Here's how the part is built. I have some questions about the finished solid (model axes, mm). A direction names the side the tool comes from. Coordinates: 2 decimals unless noted, no trailing zeros. Write each loop counter-clockwise with the first axis right and the second up, starting at its lowest first coordinate (ties: lowest second). Pieces come first, ordered by that corner, then holes.
Item 1: If we section it at C-C (y = 73.5): Please give me the cut outline in (x, z), then the cut area to 3 significant figures.
Item 2: If we section it at D-D (y = -6): Please give me the cut outline in (x, z).
Item 3: For faces 5 (the face through (30, 36, 19)), 6 (the face through (13, 52, 19)), 7 (the face through (39.067, 73.541, 13.648)), which set-ups out of +Z, -Z, +X, -X, +Y, -Y let a thin tool reach every point of the face, with its end or its side?
Item 4: I'm going to push flat-ended pins straight in: pin 1 Ø5 at (y, z) = (34, 17.5) entering from -X; pin 2 Ø4 at (x, z) = (38, 19.5) entering from -Y; pin 3 Ø6 at (x, y) = (39, 5.5) entering from -Z. Where does each tip first touch, or does it pass through?
Item 5: If I drill on line 1 (Y direction, x = 33, z = 15); line 2 (Y direction, x = 52.4, z = 18); line 3 (X direction, y = 70.5, z = 9.5), over which ranges is the centre line in solid material (lowest first)?
Item 6: If we section it at B-B (z = 19.75): Count the separate pieces of the cut face and the enclosed holes in it, then the cut area to 3 significant figures.
Item 7: If we section it at A-A (y = 39.5): Please give me the cut outline in (x, z).
Item 8: We'd pull the mould along Y, two halves only. Please class faces 1 (the face through (15, -19, 19)), 2 (the face through (20, 53.43, 18.7)), 3 (the face through (30, -15, 19)), 4 (the face through (35.85, 73, 11)): +Y half, -Y half, draft (parallel to the pull), parting line (faces both ways), or undercut.
from build123d import *

# Parameters (mm, degrees)
SKETCH1_R           = 4
SKETCH1_W           = 10.5
SKETCH1_H           = 11.5
BOSS_EXTRUDE1_DEPTH = 22
CUT_EXTRUDE1_DEPTH  = 14
SKETCH5_W           = 17
SKETCH5_H           = 15.5
SKETCH5_R           = 2.9
CUT_EXTRUDE2_DEPTH  = 2.1
CUT_EXTRUDE3_START  = -2.1
SKETCH4_W           = 17
SKETCH4_H           = 15.5
SKETCH4_R           = 2.9
CUT_EXTRUDE3_DEPTH  = 2.1
CUT_EXTRUDE4_START  = -16.1
CUT_EXTRUDE4_DEPTH  = 14
CUT_EXTRUDE5_DEPTH  = 14
CUT_EXTRUDE6_REACH  = 138.799
CUT_EXTRUDE8_DEPTH  = 1.5


with BuildPart() as part:
    # Sketch1 → Boss-Extrude1 (new body)
    with BuildSketch(Plane.XY):
        with BuildLine():
            Line((0, 13.076696831), (0, 42))
            ThreePointArc((0, 42), (2.928932188, 49.071067812), (10, 52))
            Line((10, 52), (16.5, 52))
            ThreePointArc((16.5, 52), (20.035533906, 53.464466094), (21.5, 57))
            Line((21.5, 57), (21.5, 81.25))
            Line((21.5, 81.25), (39.7, 81.25))
            Line((39.7, 81.25), (39.7, 61.75))
            Line((39.7, 61.75), (35, 61.75))
            ThreePointArc((35, 61.75), (31.464466094, 60.285533906), (30, 56.75))
            Line((30, 56.75), (30, 14))
            ThreePointArc((30, 14), (31.464466094, 10.464466094), (35, 9))
            Line((35, 9), (52.4, 9))
            ThreePointArc((52.4, 9), (61.4, 0), (52.4, -9))
            Line((52.4, -9), (35, -9))
            ThreePointArc((35, -9), (31.464466094, -10.464466094), (30, -14))
            Line((30, -14), (30, -17))
            ThreePointArc((30, -17), (27.071067812, -24.071067812), (20, -27))
            Line((20, -27), (12, -27))
            ThreePointArc((12, -27), (8.464466094, -28.464466094), (7, -32))
            Line((7, -32), (7, -39))
            Line((7, -39), (-9, -39))
            Line((-9, -39), (-9, 0))
            ThreePointArc((-9, 0), (-7.413790239, 5.102520386), (-3.214285714, 8.406447963))
            ThreePointArc((-3.214285714, 8.406447963), (-0.881227645, 10.241963283), (0, 13.076696831))
        make_face()
        Circle(SKETCH1_R, mode=Mode.SUBTRACT)
        with Locations((52.4, 0)):
            Circle(SKETCH1_R, mode=Mode.SUBTRACT)
        with BuildLine():
            Line((42.5, -2.5), (26.5, -2.5))
            ThreePointArc((26.5, -2.5), (26.146446609, -2.353553391), (26, -2))
            Line((26, -2), (26, 5))
            ThreePointArc((26, 5), (26.146446609, 5.353553391), (26.5, 5.5))
            Line((26.5, 5.5), (42.5, 5.5))
            ThreePointArc((42.5, 5.5), (42.853553391, 5.353553391), (43, 5))
            Line((43, 5), (43, -2))
            ThreePointArc((43, -2), (42.853553391, -2.353553391), (42.5, -2.5))
        make_face(mode=Mode.SUBTRACT)
        with BuildLine():
            Line((8, 42), (8, -17))
            ThreePointArc((8, -17), (8.585786438, -18.414213562), (10, -19))
            Line((10, -19), (20, -19))
            ThreePointArc((20, -19), (21.414213562, -18.414213562), (22, -17))
            Line((22, -17), (22, 42))
            ThreePointArc((22, 42), (21.414213562, 43.414213562), (20, 44))
            Line((20, 44), (10, 44))
            ThreePointArc((10, 44), (8.585786438, 43.414213562), (8, 42))
        make_face(mode=Mode.SUBTRACT)
        with Locations((30.6, 73.5)):
            Rectangle(SKETCH1_W, SKETCH1_H, mode=Mode.SUBTRACT)
    extrude(amount=BOSS_EXTRUDE1_DEPTH)

    # Sketch3 → Cut-Extrude1 (cut)
    with BuildSketch(Plane(origin=(0, 0, 0), x_dir=(-1, 0, 0), z_dir=(0, 0, -1))):
        with BuildLine():
            Line((-21.5, 61.75), (-35, 61.75))
            ThreePointArc((-35, 61.75), (-31.464466094, 60.285533906), (-30, 56.75))
            Line((-30, 56.75), (-30, 14))
            ThreePointArc((-30, 14), (-31.464466094, 10.464466094), (-35, 9))
            Line((-35, 9), (-52.4, 9))
            ThreePointArc((-52.4, 9), (-61.4, 0), (-52.4, -9))
            Line((-52.4, -9), (-35, -9))
            ThreePointArc((-35, -9), (-31.464466094, -10.464466094), (-30, -14))
            Line((-30, -14), (-30, -17))
            ThreePointArc((-30, -17), (-27.071067812, -24.071067812), (-20, -27))
            Line((-20, -27), (-12, -27))
            ThreePointArc((-12, -27), (-8.464466094, -28.464466094), (-7, -32))
            Line((-7, -32), (-7, -23.75))
            Line((-7, -23.75), (9, -23.75))
            Line((9, -23.75), (9, 0))
            ThreePointArc((9, 0), (7.413790239, 5.102520386), (3.214285714, 8.406447963))
            ThreePointArc((3.214285714, 8.406447963), (0.881227645, 10.241963283), (0, 13.076696831))
            Line((0, 13.076696831), (0, 42))
            ThreePointArc((0, 42), (-2.928932188, 49.071067812), (-10, 52))
            Line((-10, 52), (-16.5, 52))
            ThreePointArc((-16.5, 52), (-20.035533906, 53.464466094), (-21.5, 57))
            Line((-21.5, 57), (-21.5, 61.75))
        make_face()
    extrude(amount=-CUT_EXTRUDE1_DEPTH, mode=Mode.SUBTRACT)

    # Sketch5 → Cut-Extrude2 (cut)
    with BuildSketch(Plane.ZY.offset(-21.5)):
        with Locations((13.5, 73.5)):
            Rectangle(SKETCH5_W, SKETCH5_H)
        with Locations(Location((12.5, 73.5, 0), (0, 0, 90))):
            Circle(SKETCH5_R, mode=Mode.SUBTRACT)
    extrude(amount=-CUT_EXTRUDE2_DEPTH, mode=Mode.SUBTRACT)

    # Sketch4 → Cut-Extrude3 (cut)
    with BuildSketch(Plane(origin=(39.7, 0, 0), x_dir=(0, 0, -1), z_dir=(1, 0, 0)).offset(CUT_EXTRUDE3_START)):
        with Locations((-13.5, 73.5)):
            Rectangle(SKETCH4_W, SKETCH4_H)
        with Locations(Location((-12.5, 73.5, 0), (0, 0, 90))):
            Circle(SKETCH4_R, mode=Mode.SUBTRACT)
    extrude(amount=CUT_EXTRUDE3_DEPTH, mode=Mode.SUBTRACT)

    # Sketch6 → Cut-Extrude4 (cut)
    with BuildSketch(Plane.ZY.offset(-21.5).offset(CUT_EXTRUDE4_START)):
        Polygon((12.5, 81.25), (14.5, 79.25), (22, 79.25), (22, 81.25), align=None)
        Polygon((12.5, 65.75), (14.5, 67.75), (22, 67.75), (22, 65.75), align=None)
    extrude(amount=CUT_EXTRUDE4_DEPTH, mode=Mode.SUBTRACT)

    # Sketch7 → Cut-Extrude5 (cut)
    with BuildSketch(Plane.XY.offset(22)):
        Polygon((25.35, 81.25), (35.85, 81.25), (35.85, 65.75), (39.7, 65.75), (39.7, 65.25), (21.5, 65.25), (21.5, 65.75), (25.35, 65.75), align=None)
    extrude(amount=-CUT_EXTRUDE5_DEPTH, mode=Mode.SUBTRACT)

    # Cut-Extrude6: up to this face of the body (flat: up to its plane)
    cut_extrude6_end = Plane(part.part.faces().sort_by_distance((22.55, 65.75, 6.5))[0])
    # Sketch8 → Cut-Extrude6 (cut, up to the picked face)
    with BuildSketch(Plane(origin=(0, 81.25, 0), x_dir=(1, 0, 0), z_dir=(0, 1, 0)), mode=Mode.PRIVATE) as cut_extrude6_sk1:
        Polygon((21.5, -12.5), (23.1, -15.4), (21.5, -15.4), align=None)
    cut_extrude6_tool1 = split(extrude(cut_extrude6_sk1.sketch, amount=-CUT_EXTRUDE6_REACH, mode=Mode.PRIVATE), bisect_by=cut_extrude6_end, keep=Keep.BOTH, mode=Mode.PRIVATE)
    # Sketch8 → Cut-Extrude6 (cut, up to the picked face)
    with BuildSketch(Plane(origin=(0, 81.25, 0), x_dir=(1, 0, 0), z_dir=(0, 1, 0)), mode=Mode.PRIVATE) as cut_extrude6_sk2:
        Polygon((39.7, -15.4), (38.1, -15.4), (39.7, -12.5), align=None)
    cut_extrude6_tool2 = split(extrude(cut_extrude6_sk2.sketch, amount=-CUT_EXTRUDE6_REACH, mode=Mode.PRIVATE), bisect_by=cut_extrude6_end, keep=Keep.BOTH, mode=Mode.PRIVATE)
    add(cut_extrude6_tool1.solids().sort_by(Axis((22.033333, 81.25, 14.433333), (0, -1, 0)))[0], mode=Mode.SUBTRACT)
    add(cut_extrude6_tool2.solids().sort_by(Axis((39.166667, 81.25, 14.433333), (0, -1, 0)))[0], mode=Mode.SUBTRACT)

    # Sketch10 → Cut-Extrude8 (cut)
    with BuildSketch(Plane(origin=(0, 0, 14), x_dir=(-1, 0, 0), z_dir=(0, 0, -1))):
        with BuildLine():
            Line((-35, 9), (2.105083257, 9))
            ThreePointArc((2.105083257, 9), (0.557332799, 10.782637515), (0, 13.076696831))
            Line((0, 13.076696831), (0, 42))
            ThreePointArc((0, 42), (-2.928932188, 49.071067812), (-10, 52))
            Line((-10, 52), (-16.5, 52))
            ThreePointArc((-16.5, 52), (-20.035533906, 53.464466094), (-21.5, 57))
            Line((-21.5, 57), (-21.5, 61.75))
            Line((-21.5, 61.75), (-35, 61.75))
            ThreePointArc((-35, 61.75), (-31.464466094, 60.285533906), (-30, 56.75))
            Line((-30, 56.75), (-30, 14))
            ThreePointArc((-30, 14), (-31.464466094, 10.464466094), (-35, 9))
        make_face()
        with BuildLine():
            Line((-35, -9), (0, -9))
            ThreePointArc((0, -9), (6.363961031, -6.363961031), (9, 0))
            Line((9, 0), (9, -23.75))
            Line((9, -23.75), (-7, -23.75))
            Line((-7, -23.75), (-7, -32))
            ThreePointArc((-7, -32), (-8.464466094, -28.464466094), (-12, -27))
            Line((-12, -27), (-20, -27))
            ThreePointArc((-20, -27), (-27.071067812, -24.071067812), (-30, -17))
            Line((-30, -17), (-30, -14))
            ThreePointArc((-30, -14), (-31.464466094, -10.464466094), (-35, -9))
        make_face()
    extrude(amount=-CUT_EXTRUDE8_DEPTH, mode=Mode.SUBTRACT)


solid = part.part
Answer list:
1. outline: (21.5, 0) - (25.35, 0) - (25.35, 22) - (23.6, 22) - (23.6, 15.4) - (23.1, 15.4) - (21.5, 12.5) - (21.5, 9.6) - (23.6, 9.6) - (23.6, 5) - (21.5, 5) - close; (35.85, 0) - (39.7, 0) - (39.7, 5) - (37.6, 5) - (37.6, 9.6) - (39.7, 9.6) - (39.7, 12.5) - (38.1, 15.4) - (37.6, 15.4) - (37.6, 22) - (35.85, 22) - close
1. area: 118 mm2
2. outline: (-9, 15.5) - (-6.71, 15.5) - (-6.71, 14) - (8, 14) - (8, 22) - (-9, 22) - close; (22, 14) - (59.11, 14) - (59.11, 22) - (22, 22) - close
3. face 5: +Z, -Z, +X
3. face 6: +Z, -Z, -X, +Y
3. face 7: +Z, +X, +Y
4. pin 1: stops at x = 0
4. pin 2: stops at y = -9
4. pin 3: stops at z = 14
5. line 1: y = -9 to -2.5, 5.5 to 9, 61.75 to 65.25
5. line 2: y = -9 to -4, 4 to 9
5. line 3: x = 23.6 to 25.35, 35.85 to 37.6
6. separate pieces: 3
6. enclosed holes: 4
6. area: 2,460 mm2
7. outline: (0, 15.5) - (8, 15.5) - (8, 22) - (0, 22) - close; (22, 15.5) - (30, 15.5) - (30, 22) - (22, 22) - close
8. face 1: undercut
8. face 2: +Y half
8. face 3: draft
8. face 4: undercut
